Can you work these out from the model? Positions are in its coordinate system, mm. Face numbers are marked on the shaded views. A direction names the side the tool comes from. Give positions to 0.01 mm unless a question says otherwise; leave off trailing zeros. Order: outer loops, then holes, each group sorted by start corner. A loop starts at its lowest first (then second) coordinate and runs counter-clockwise, first axis right, second up. Notation, with made-up numbers: M 82.5,85 L 138.5,85 A21 ccw 138.5,100 Z; hole C 85,42 d9. An arc over 180 degrees is marked long. Answer as a JSON object with one key per item and string values.
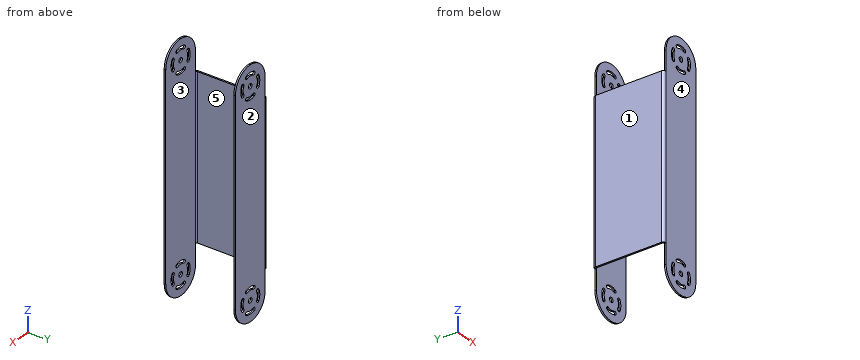
```python
from build123d import *

# Parameters (mm, degrees)
SKETCH_1_W             = 25
SKETCH_1_H             = 100
SM_BASE_FLANGE_1_DEPTH = 1
SM_EDGE_FLANGE_1_DEPTH = 100
SM_EDGE_FLANGE_2_DEPTH = 100
SKETCH_18_W            = 25
SKETCH_18_H            = 1
EXTRUDE_1_DEPTH        = 25
FILLET_1_R             = 12.5
SKETCH_21_R            = 1.5
CUT_EXTRUDE_1_DEPTH    = 89.735735525
FILLET_1_OF_MIRROR_1_R = 12.5


# Sheet-metal steps are written as plain solids
with BuildPart() as part:
    # Sketch 1 → 基材-凸緣1 (new body)
    with BuildSketch(Plane(origin=(0, 0, 0), x_dir=(1, 0, 0), z_dir=(0, 1, 0))):
        Rectangle(SKETCH_1_W, SKETCH_1_H)
    extrude(amount=-SM_BASE_FLANGE_1_DEPTH)

    # 邊線-凸緣1 section (across the edge) → 邊線-凸緣1 (add)
    with BuildSketch(Plane(origin=(-13.2366, -1, 50), x_dir=(1, 0, 0), z_dir=(0, 0, -1))):
        with BuildLine():
            Line((-1, 0.7366), (-1, 42.5))
            Line((-1, 42.5), (0, 42.5))
            Line((0, 42.5), (0, 0.7366))
            ThreePointArc((0, 0.7366), (0.215745145, 0.215745145), (0.7366, 0))
            Line((0.7366, 0), (0.7366, -1))
            ThreePointArc((0.7366, -1), (-0.491361636, -0.491361636), (-1, 0.7366))
        make_face()
    extrude(amount=SM_EDGE_FLANGE_1_DEPTH)

    # 邊線-凸緣2 section (across the edge) → 邊線-凸緣2 (add)
    with BuildSketch(Plane(origin=(-13.2366, -44.2366, 50), x_dir=(0, 1, 0), z_dir=(0, 0, -1))):
        with BuildLine():
            Line((-1, 0.7366), (-1, 25.7366))
            Line((-1, 25.7366), (0, 25.7366))
            Line((0, 25.7366), (0, 0.7366))
            ThreePointArc((0, 0.7366), (0.215745145, 0.215745145), (0.7366, 0))
            Line((0.7366, 0), (0.7366, -1))
            ThreePointArc((0.7366, -1), (-0.491361636, -0.491361636), (-1, 0.7366))
        make_face()
    extrude(amount=SM_EDGE_FLANGE_2_DEPTH)

    # 草圖18 → 填料-伸長1 (add)
    with BuildSketch(Plane.XY.offset(50)):
        with Locations((0, -0.5)):
            Rectangle(SKETCH_18_W, SKETCH_18_H)
        with Locations((0, -44.7366)):
            Rectangle(SKETCH_18_W, SKETCH_18_H)
    extrude_1 = extrude(amount=EXTRUDE_1_DEPTH)

    # 圓角1
    fillet_1_edges = [part.edges().sort_by_distance(p)[0] for p in [
        (-12.5, -44.7366, 75),
        (12.5, -44.7366, 75),
        (12.5, -0.5, 75),
        (-12.5, -0.5, 75),
    ]]
    fillet(fillet_1_edges, radius=FILLET_1_R - 0.0001)  # a hair under: the kernel refuses the full size

    # 草圖21 → 除料-伸長1 (cut, through all)
    with BuildSketch(Plane(origin=(0, 0, 0), x_dir=(1, 0, 0), z_dir=(0, 1, 0))):
        with Locations(Location((0, -62.5, 0), (0, 0, 270))):
            Circle(SKETCH_21_R)
        with BuildLine():
            ThreePointArc((3.428571429, -55.271936777), (0, -54.5), (-3.428571429, -55.271936777))
            ThreePointArc((-3.428571429, -55.271936777), (-3.903507903, -56.604016108), (-2.571428571, -57.078952583))
            ThreePointArc((-2.571428571, -57.078952583), (0, -56.5), (2.571428571, -57.078952583))
            ThreePointArc((2.571428571, -57.078952583), (3.903507903, -56.604016108), (3.428571429, -55.271936777))
        make_face()
        with BuildLine():
            ThreePointArc((5.421047417, -65.071428571), (6, -62.5), (5.421047417, -59.928571429))
            ThreePointArc((5.421047417, -59.928571429), (5.895983892, -58.596492097), (7.228063223, -59.071428571))
            ThreePointArc((7.228063223, -59.071428571), (8, -62.5), (7.228063223, -65.928571429))
            ThreePointArc((7.228063223, -65.928571429), (5.895983892, -66.403507903), (5.421047417, -65.071428571))
        make_face()
        with BuildLine():
            ThreePointArc((-2.571428571, -67.921047417), (0, -68.5), (2.571428571, -67.921047417))
            ThreePointArc((2.571428571, -67.921047417), (3.903507903, -68.395983892), (3.428571429, -69.728063223))
            ThreePointArc((3.428571429, -69.728063223), (0, -70.5), (-3.428571429, -69.728063223))
            ThreePointArc((-3.428571429, -69.728063223), (-3.903507903, -68.395983892), (-2.571428571, -67.921047417))
        make_face()
        with BuildLine():
            ThreePointArc((-5.421047417, -59.928571429), (-6, -62.5), (-5.421047417, -65.071428571))
            ThreePointArc((-5.421047417, -65.071428571), (-5.895983892, -66.403507903), (-7.228063223, -65.928571429))
            ThreePointArc((-7.228063223, -65.928571429), (-8, -62.5), (-7.228063223, -59.071428571))
            ThreePointArc((-7.228063223, -59.071428571), (-5.895983892, -58.596492097), (-5.421047417, -59.928571429))
        make_face()
    cut_extrude_1 = extrude(amount=-CUT_EXTRUDE_1_DEPTH, mode=Mode.SUBTRACT)

    # 鏡射1: 填料-伸長1, 除料-伸長1 across plane
    add(extrude_1.mirror(Plane.XY))
    add(cut_extrude_1.mirror(Plane.XY), mode=Mode.SUBTRACT)

    # 圓角1 of 鏡射1
    fillet_1_of_mirror_1_edges = [part.edges().sort_by_distance(p)[0] for p in [
        (-12.5, -44.7366, -75),
        (12.5, -44.7366, -75),
        (12.5, -0.5, -75),
        (-12.5, -0.5, -75),
    ]]
    fillet(fillet_1_of_mirror_1_edges, radius=FILLET_1_OF_MIRROR_1_R - 0.0001)  # a hair under: the kernel refuses the full size


solid = part.part
```
1) I want a section at B-B on z = 32.5. Write out the boundary of the cut face in (x, y), and give its area (3 significant figures).
Results found:
{"outline": "M -14.24,-43.5 A1.74 ccw -12.5,-45.24 L 12.5,-45.24 L 12.5,-44.24 L -12.5,-44.24 A0.74 cw -13.24,-43.5 L -13.24,-1.74 A0.74 cw -12.5,-1 L 12.5,-1 L 12.5,0 L -12.5,0 A1.74 ccw -14.24,-1.74 Z", "area": "95.6 mm²"}
2) I want a section at C-C on y = -28.5. Write out the boundary of the cut face in (x, z).
Results found:
{"outline": "M -14.24,-50 L -13.24,-50 L -13.24,50 L -14.24,50 Z"}
3) For the marked faces 4 and 5, which set-ups out of +Z, -Z, +X, -X, +Y, -Y let a thin tool reach every point of the face, with its end or its side?
Results found:
{"face 4": "+Z, -Z, +X, -X, -Y", "face 5": "+Z, -Z, +X"}
4) Thinking about a two-plate mould opening in Y: for the marked faces 1, 2 and 3, which applies, pulls with the +Y half, pulls with the -Y half, needs draft (parallel to the pull), parting line crosses it, or undercut?
Results found:
{"face 1": "needs draft", "face 2": "pulls with the +Y half", "face 3": "undercut"}
5) I want a section at A-A on x = 10. Write out the boundary of the cut face in (y, z), and give its area (3 significant figures).
Results found:
{"outline": "M -45.24,-70 L -44.24,-70 L -44.24,70 L -45.24,70 Z; M -1,-70 L 0,-70 L 0,70 L -1,70 Z", "area": "280 mm²"}
6) I need wall thicknesses on L1, parallel to X at y = -0.6, z = 62.5; L2, parallel to Y at x = 8.5, z = -41; L3, parallel to X at y = -7.5, z = 2. Which ranges of each line are inside material? Lowest first, please.
Results found:
{"L1": "x = -12.5 to -8, -6 to -1.5, 1.5 to 6, 8 to 12.5", "L2": "y = -45.24 to -44.24, -1 to 0", "L3": "x = -14.24 to -13.24"}
7) I'm going to push flat-ended pins straight in: pin 1 Ø1.9 at (x, y) = (-13.5, -26.5) entering from -Z; pin 2 Ø1.4 at (x, y) = (-13, -26) entering from +Z; pin 3 Ø10 at (y, z) = (-35.5, 24) entering from +X; pin 4 Ø2.5 at (x, z) = (0, 62.5) entering from +Y. Where does each tip first touch, or does it pass through?
Results found:
{"pin 1": "stops at z = -50", "pin 2": "stops at z = 50", "pin 3": "stops at x = -13.24", "pin 4": "passes through"}
